Could you check a few things on this model? Use its own coordinates, in mm. Give positions to 0.01 mm unless a question says otherwise; leave off trailing zeros. Return JSON: item names as keys, results as strings. Group by question number.
```python
from build123d import *

# Parameters (mm, degrees)
SKETCH_1_W             = 55
SKETCH_1_H             = 780
EXTRUDE_1_DEPTH        = 3
CUT_EXTRUDE_1_DEPTH    = 7
HOLE_WIZARD_M6_1_D     = 5
HOLE_WIZARD_M6_1_DEPTH = 17
HOLE_WIZARD_M6_1_TIP   = 1.502151548


with BuildPart() as part:
    # 草图1 → 凸台-拉伸1 (new body, symmetric)
    with BuildSketch(Plane.XY):
        Rectangle(SKETCH_1_W, SKETCH_1_H)
    extrude(amount=EXTRUDE_1_DEPTH, both=True)

    # 草图4 → 切除-拉伸1 (cut, through all)
    with BuildSketch(Plane(origin=(0, 0, -3), x_dir=(-1, 0, 0), z_dir=(0, 0, -1))):
        with BuildLine():
            Line((3.251986045, -21.579414933), (-2.748013955, -21.579414933))
            ThreePointArc((-2.748013955, -21.579414933), (-4.162227517, -20.993628496), (-4.748013955, -19.579414933))
            Line((-4.748013955, -19.579414933), (-4.748013955, 6.420585067))
            ThreePointArc((-4.748013955, 6.420585067), (-4.162227517, 7.834798629), (-2.748013955, 8.420585067))
            Line((-2.748013955, 8.420585067), (3.251986045, 8.420585067))
            ThreePointArc((3.251986045, 8.420585067), (4.666199608, 7.834798629), (5.251986045, 6.420585067))
            Line((5.251986045, 6.420585067), (5.251986045, -19.579414933))
            ThreePointArc((5.251986045, -19.579414933), (4.666199608, -20.993628496), (3.251986045, -21.579414933))
        make_face()
    extrude(amount=-CUT_EXTRUDE_1_DEPTH, mode=Mode.SUBTRACT)

    # M6 螺纹孔1
    with Locations(Plane(origin=(0, 0, -3), x_dir=(-1, 0, 0), z_dir=(0, 0, -1))):
        with Locations((20, 302), (-20, 302), (20, -236), (-20, -236)):
            Hole(HOLE_WIZARD_M6_1_D / 2, depth=HOLE_WIZARD_M6_1_DEPTH)
            with Locations((0, 0, -(HOLE_WIZARD_M6_1_DEPTH + HOLE_WIZARD_M6_1_TIP / 2))):  # 118° drill point
                Cone(0, HOLE_WIZARD_M6_1_D / 2, HOLE_WIZARD_M6_1_TIP, mode=Mode.SUBTRACT)


solid = part.part
```
1. I need wall thicknesses on L1, parallel to X at y = -236, z = -1.5; L2, parallel to Y at x = 20, z = 0.3; L3, parallel to Y at x = 20.5, z = -1.05. Which ranges of each line are inside material? Lowest first, please. Write a range as from..to.
2. For pin 1 (4.5 mm diameter, centred on x = -20, y = 302, fed in from -Z), with a flat end and sliding along its axis, tell me the tip position at first contact or that it passes through.
3. If we mould it in two halves opening along Z, with no side actions, what happens to faces 1 (the flat face through (-6, 5, 3)), 2 (the flat face through (-6, 5, -3))? For each: pulls with the +Z half, pulls with the -Z half, needs draft (parallel to the pull), parting line crosses it, or undercut.
Values:
{
 "1": {"L1": "x = -27.5..-22.5, -17.5..17.5, 22.5..27.5", "L2": "y = -390..-238.5, -233.5..299.5, 304.5..390", "L3": "y = -390..-238.45, -233.55..299.55, 304.45..390"},
 "2": {"pin 1": "passes through"},
 "3": {"face 1": "pulls with the +Z half", "face 2": "pulls with the -Z half"}
}
